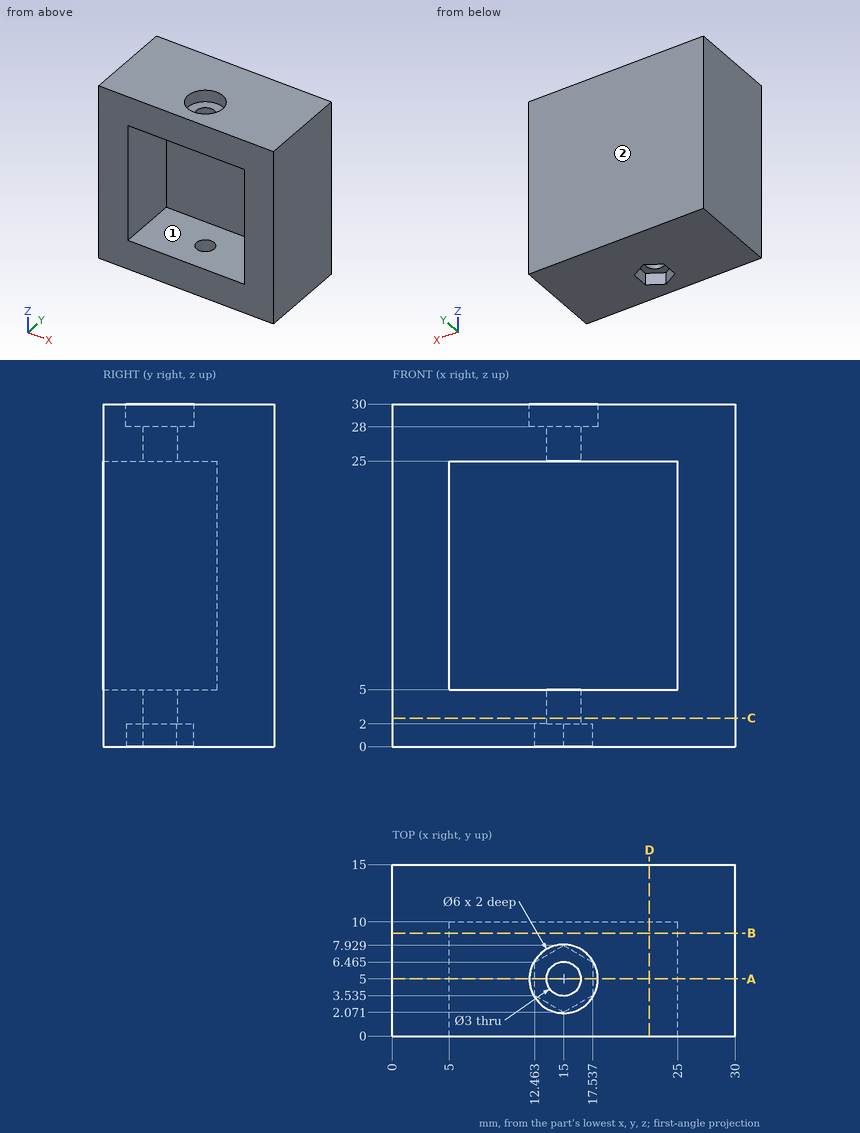
Can you work these out from the drawing? Everything is in mm from the part's minimum corner. A direction names the side the tool comes from. Round coordinates to 2 decimals unless told otherwise and drop trailing zeros. Loops run counter-clockwise (first coordinate to the right, second up) from the corner with the lowest first, then second, coordinate; pieces in that order, holes last. Notation, with made-up numbers: (55, 31) - (76, 31) arc R23 ccw to (76, 60) - close; hole circle Ø8 at (76, 4). An arc over 180 degrees is marked (long way). Answer in a Markdown table with one row per item. Add a question column.
Q1. I want a section at C-C on z = 2.5. List the corners of the cut face in (x, y) for me.
Q2. For pin 1 Ø1.8 at (x, y) = (15, 5) entering from +Z; pin 2 Ø1.5 at (x, y) = (13, 5.5) entering from +Z, each with a flat end and sliding along its axis, tell me the tip position at first contact or that it passes through.
Q3. I want a section at B-B on y = 9. List the corners of the cut face in (x, z) for me, and give its area (3 significant figures).
Q4. I want a section at A-A on y = 5. List the corners of the cut face in (x, z) for me, and give its area (3 significant figures).
Q5. I need wall thicknesses on L1, parallel to Y at x = 15, z = 27.4; L2, parallel to X at y = 2.5, z = 10; L3, parallel to Z at x = 16.5, y = 4.5. Which ranges of each line are inside material? Lowest first, please.
Q6. I want a section at D-D on x = 22.5. List the corners of the cut face in (y, z) for me.
Q7. Which directions (+Z, -Z, +X, -X, +Y, -Y) give clear straight access to the entire face, cutting with the end or side of a thin tool? Please do the marked faces 1 and 2.
A:
| question | item | result |
|---|---|---|
| 1 | outline | (0, 0) - (30, 0) - (30, 15) - (0, 15) - close; hole circle Ø3 at (15, 5) |
| 2 | pin 1 | through |
| 2 | pin 2 | z = 28 |
| 3 | outline | (0, 0) - (30, 0) - (30, 30) - (0, 30) - close; hole (5, 5) - (25, 5) - (25, 25) - (5, 25) - close |
| 3 | area | 500 mm^2 |
| 4 | outline | (0, 0) - (12.46, 0) - (12.46, 2) - (13.5, 2) - (13.5, 5) - (5, 5) - (5, 25) - (13.5, 25) - (13.5, 28) - (12, 28) - (12, 30) - (0, 30) - close; (16.5, 2) - (17.54, 2) - (17.54, 0) - (30, 0) - (30, 30) - (18, 30) - (18, 28) - (16.5, 28) - (16.5, 25) - (25, 25) - (25, 5) - (16.5, 5) - close |
| 4 | area | 460 mm^2 |
| 5 | L1 | 0 to 3.5, 6.5 to 15 |
| 5 | L2 | 0 to 5, 25 to 30 |
| 5 | L3 | 2 to 5, 25 to 28 |
| 6 | outline | (0, 0) - (15, 0) - (15, 30) - (0, 30) - (0, 25) - (10, 25) - (10, 5) - (0, 5) - close |
| 7 | face 1 | -Y |
| 7 | face 2 | +Z, -Z, +X, -X, +Y |
